Build history of the part. All positions in model axes, mm. A direction names the side the tool comes from. Give positions to 0.01 mm unless a question says otherwise; leave off trailing zeros. Write each loop counter-clockwise with the first axis right and the second up, starting at its lowest first coordinate (ties: lowest second). Pieces come first, ordered by that corner, then holes.
from build123d import *

# Parameters (mm, degrees)
SKETCH2_R           = 3.05
SKETCH2_R_2         = 2
BOSS_EXTRUDE1_DEPTH = 7
CUT_EXTRUDE1_START  = 7
SKETCH2_4_R         = 9.5
CUT_EXTRUDE1_DEPTH  = 6
CUT_EXTRUDE2_START  = 7
SKETCH2_5_R         = 6.5
CUT_EXTRUDE2_DEPTH  = 5
CUT_EXTRUDE3_DEPTH  = 4.5


with BuildPart() as part:
    # Sketch2 → Boss-Extrude1 (new body)
    with BuildSketch(Plane(origin=(0, 0, 0), x_dir=(1, 0, 0), z_dir=(0, 1, 0))):
        with BuildLine():
            Line((102.512048312, 24.992099408), (102.512048312, -23.007900592))
            Line((102.512048312, -23.007900592), (84.012048312, -23.007900592))
            Line((84.012048312, -23.007900592), (84.012048312, -15.007900592))
            Line((84.012048312, -15.007900592), (49.012048312, -15.007900592))
            Line((49.012048312, -15.007900592), (49.012048312, -23.007900592))
            Line((49.012048312, -23.007900592), (31.512048312, -23.007900592))
            Line((31.512048312, -23.007900592), (31.512048312, -13.007900592))
            Line((31.512048312, -13.007900592), (30.016072392, 39.708435169))
            ThreePointArc((30.016072392, 39.708435169), (33.741164308, 47.78158038), (42.423514406, 49.696986387))
            Line((42.423514406, 49.696986387), (93.026380929, 37.123208132))
            ThreePointArc((93.026380929, 37.123208132), (99.859107713, 32.691802074), (102.512048312, 24.992099408))
        make_face()
        with Locations(Location((90.012048312, 24.992099408, 0), (0, 0, 270))):
            Circle(SKETCH2_R, mode=Mode.SUBTRACT)
        with Locations(Location((40.012048312, 39.992099408, 0), (0, 0, 270))):
            Circle(SKETCH2_R_2, mode=Mode.SUBTRACT)
        with BuildLine():
            Line((51.378851017, 18.833843692), (54.349655223, 19.251362995))
            ThreePointArc((54.349655223, 19.251362995), (67.338228674, 9.463770865), (57.550636545, -3.524802586))
            Line((57.550636545, -3.524802586), (54.579832339, -3.942321889))
            ThreePointArc((54.579832339, -3.942321889), (41.591258887, 5.84527024), (51.378851017, 18.833843692))
        make_face(mode=Mode.SUBTRACT)
        with BuildLine():
            Line((65.962554027, 26.437501135), (68.933358233, 26.855020438))
            ThreePointArc((68.933358233, 26.855020438), (70.627519988, 25.578377986), (69.350877536, 23.884216232))
            Line((69.350877536, 23.884216232), (66.38007333, 23.466696929))
            ThreePointArc((66.38007333, 23.466696929), (64.685911575, 24.74333938), (65.962554027, 26.437501135))
        make_face(mode=Mode.SUBTRACT)
        with BuildLine():
            Line((70.694439459, -7.231613202), (73.665243666, -6.814093899))
            ThreePointArc((73.665243666, -6.814093899), (74.941886117, -5.119932145), (73.247724363, -3.843289693))
            Line((73.247724363, -3.843289693), (70.276920157, -4.260808996))
            ThreePointArc((70.276920157, -4.260808996), (69.000277705, -5.954970751), (70.694439459, -7.231613202))
        make_face(mode=Mode.SUBTRACT)
        with BuildLine():
            Line((42.966933535, -11.128460029), (39.996129329, -11.545979332))
            ThreePointArc((39.996129329, -11.545979332), (38.301967574, -10.26933688), (39.578610026, -8.575175126))
            Line((39.578610026, -8.575175126), (42.549414232, -8.157655823))
            ThreePointArc((42.549414232, -8.157655823), (44.243575986, -9.434298275), (42.966933535, -11.128460029))
        make_face(mode=Mode.SUBTRACT)
        with BuildLine():
            Line((38.235048102, 22.540654308), (35.264243896, 22.123135005))
            ThreePointArc((35.264243896, 22.123135005), (33.987601444, 20.428973251), (35.681763199, 19.152330799))
            Line((35.681763199, 19.152330799), (38.652567405, 19.569850102))
            ThreePointArc((38.652567405, 19.569850102), (39.929209857, 21.264011856), (38.235048102, 22.540654308))
        make_face(mode=Mode.SUBTRACT)
    extrude(amount=BOSS_EXTRUDE1_DEPTH)

    # Sketch2<4> → Cut-Extrude1 (cut)
    with BuildSketch(Plane(origin=(0, 0, 0), x_dir=(1, 0, 0), z_dir=(0, 1, 0)).offset(CUT_EXTRUDE1_START)):
        with Locations(Location((90.012048312, 24.992099408, 0), (0, 0, 270))):
            Circle(SKETCH2_4_R)
    extrude(amount=-CUT_EXTRUDE1_DEPTH, mode=Mode.SUBTRACT)

    # Sketch2<5> → Cut-Extrude2 (cut)
    with BuildSketch(Plane(origin=(0, 0, 0), x_dir=(1, 0, 0), z_dir=(0, 1, 0)).offset(CUT_EXTRUDE2_START)):
        with Locations(Location((40.012048312, 39.992099408, 0), (0, 0, 270))):
            Circle(SKETCH2_5_R)
    extrude(amount=-CUT_EXTRUDE2_DEPTH, mode=Mode.SUBTRACT)

    # Sketch2<6> → Cut-Extrude3 (cut)
    with BuildSketch(Plane(origin=(0, 0, 0), x_dir=(1, 0, 0), z_dir=(0, 1, 0))):
        with BuildLine():
            Line((65.788587651, 27.675336221), (68.759391857, 28.092855524))
            ThreePointArc((68.759391857, 28.092855524), (71.865355074, 25.752344362), (69.524843912, 22.646381146))
            Line((69.524843912, 22.646381146), (66.554039706, 22.228861843))
            ThreePointArc((66.554039706, 22.228861843), (63.448076489, 24.569373004), (65.788587651, 27.675336221))
        make_face()
        with BuildLine():
            Line((70.868405836, -8.469448288), (73.839210042, -8.051928985))
            ThreePointArc((73.839210042, -8.051928985), (76.179721203, -4.945965769), (73.073757987, -2.605454607))
            Line((73.073757987, -2.605454607), (70.10295378, -3.02297391))
            ThreePointArc((70.10295378, -3.02297391), (67.762442619, -6.128937127), (70.868405836, -8.469448288))
        make_face()
        with BuildLine():
            Line((38.061081726, 23.778489394), (35.09027752, 23.360970091))
            ThreePointArc((35.09027752, 23.360970091), (32.749766358, 20.255006874), (35.855729575, 17.914495713))
            Line((35.855729575, 17.914495713), (38.826533781, 18.332015016))
            ThreePointArc((38.826533781, 18.332015016), (41.167044943, 21.437978232), (38.061081726, 23.778489394))
        make_face()
        with BuildLine():
            Line((42.375447856, -6.919820737), (39.404643649, -7.33734004))
            ThreePointArc((39.404643649, -7.33734004), (37.064132488, -10.443303257), (40.170095705, -12.783814418))
            Line((40.170095705, -12.783814418), (43.140899911, -12.366295115))
            ThreePointArc((43.140899911, -12.366295115), (45.481411072, -9.260331898), (42.375447856, -6.919820737))
        make_face()
    extrude(amount=CUT_EXTRUDE3_DEPTH, mode=Mode.SUBTRACT)


solid = part.part
(1) Probe line 1 (X direction, y = 6, z = 17); line 2 (Z direction, x = 65.5, y = 1.75); line 3 (Z direction, x = 38, y = 2.25). List the from-to ranges inside material, lowest first.
(2) 3-axis set-ups, long thin cutter, end or side, ignore diameter. For faces 1 (the face through (76.187, 2.218, 5.006)), 2 (the face through (67, 3, 15.008)), 3 (the face through (67.89, 5.73, -23.68)), 4 (the face through (99.43, 4.04, -26.23)): which of +Z, -Z, +X, -X, +Y, -Y reach the whole face in a straight line?
(3) Mould opens along X. For faces 5 (the face through (67.37, 3.45, -43.5)), 6 (the face through (41.175, 2.218, -21.378)) say: +X half, -X half, draft (parallel to the pull), parting line (faces both ways), or undercut.
(4) Saw through at C-C, the plane x = 88. List the corners of the cut face in (y, z).
(5) Drop flat-ended pins along their axis: pin 1 (1.8 mm diameter, centred on x = 36.5, z = -22, fed in from -Y); pin 2 (2 mm diameter, centred on y = 4.5, z = 19, fed in from -X); pin 3 (4 mm diameter, centred on x = 75.5, y = 5, fed in from +Z). Give the stop position or say it passes through.
(6) Saw through at A-A, the plane z = 16. List the corners of the cut face in (x, y), plus the area to 3 significant figures.
(7) Saw through at D-D, the plane z = -3. List the corners of the cut face in (x, y), plus the area to 3 significant figures.
(8) Saw through at B-B, the plane y = 6. Give the number of separate pieces and of enclosed holes in the cut face, plus the area to 3 significant figures.
Computed values:
1. line 1: x = 31.51 to 49.01, 84.01 to 102.51
1. line 2: z = -43.96 to -27.62, -22.29 to -14.27, -1.46 to 15.01
1. line 3: z = -49.79 to -46.17, -33.81 to -23.77, -18.22 to 7.97, 12.15 to 23.01
2. face 1: -Y
2. face 2: +Z, +Y, -Y
2. face 3: +Y, -Y
2. face 4: +Y
3. face 5: +X half
3. face 6: undercut
4. outline: (0, -38.37) - (7, -38.37) - (7, -34.28) - (1, -34.28) - (1, -27.28) - (0, -27.28) - close; (0, -22.7) - (1, -22.7) - (1, -15.71) - (7, -15.71) - (7, 23.01) - (0, 23.01) - close
5. pin 1: stops at y = 4.5
5. pin 2: stops at x = 31.51
5. pin 3: stops at z = 15.01
6. outline: (31.51, 0) - (49.01, 0) - (49.01, 7) - (31.51, 7) - close; (84.01, 0) - (102.51, 0) - (102.51, 7) - (84.01, 7) - close
6. area: 252 mm2
7. outline: (31.06, 0) - (42.37, 0) - (42.37, 7) - (31.06, 7) - close; (66.37, 0) - (102.51, 0) - (102.51, 7) - (66.37, 7) - close
7. area: 332 mm2
8. separate pieces: 1
8. enclosed holes: 7
8. area: 3,490 mm2
